```python
from build123d import *

# Parameters (mm, degrees)
SKETCH1_W          = 71
SKETCH1_H          = 7
EXTRUDE1_DEPTH     = 5.5
SKETCH2_W          = 65
SKETCH2_H          = 2.766320183
CUT_EXTRUDE1_DEPTH = 7.5
SKETCH3_W          = 63
SKETCH3_H          = 2
EXTRUDE2_DEPTH     = 5.5
SKETCH4_W          = 49.4
SKETCH4_H          = 2
SKETCH4_W_2        = 12.5
CUT_EXTRUDE2_DEPTH = 2.9
FILLET1_R          = 2
EXTRUDE3_START     = 1.955331485
EXTRUDE3_DEPTH     = 2.978778395
EXTRUDE3_START_2   = -35.5
EXTRUDE3_2_DEPTH   = 71


with BuildPart() as part:
    # Sketch1 → Extrude1 (new body)
    with BuildSketch(Plane(origin=(0, 0, 0), x_dir=(1, 0, 0), z_dir=(0, 1, 0))):
        Rectangle(SKETCH1_W, SKETCH1_H)
    extrude(amount=EXTRUDE1_DEPTH)

    # Sketch2 → Cut-Extrude1 (cut)
    with BuildSketch(Plane(origin=(0, 5.5, 0), x_dir=(-1, 0, 0), z_dir=(0, 1, 0))):
        with Locations((0, 3.383160092)):
            Rectangle(SKETCH2_W, SKETCH2_H)
    extrude(amount=-CUT_EXTRUDE1_DEPTH, mode=Mode.SUBTRACT)

    # Sketch3 → Extrude2 (add)
    with BuildSketch(Plane(origin=(0, 5.5, 0), x_dir=(-1, 0, 0), z_dir=(0, 1, 0))):
        with Locations((0, -4.5)):
            Rectangle(SKETCH3_W, SKETCH3_H)
    extrude(amount=-EXTRUDE2_DEPTH)

    # Sketch4 → Cut-Extrude2 (cut)
    with BuildSketch(Plane(origin=(0, 5.5, 0), x_dir=(-1, 0, 0), z_dir=(0, 1, 0))):
        with Locations((-6.8, -4.5)):
            Rectangle(SKETCH4_W, SKETCH4_H)
        with Locations((25.25, -4.5)):
            Rectangle(SKETCH4_W_2, SKETCH4_H)
    extrude(amount=-CUT_EXTRUDE2_DEPTH, mode=Mode.SUBTRACT)

    # Fillet1
    fillet1_edges = [part.edges().sort_by_distance(p)[0] for p in [
        (-18.45, 5.5, -5.5),
    ]]
    fillet(fillet1_edges, radius=FILLET1_R)

    # Extrude3: read off the stored shape, not the designer's step
    # Extrude3 outline → Extrude3 (cut)
    with BuildSketch(Plane(origin=(0, 0, 0), x_dir=(1, 0, 0), z_dir=(0, 1, 0)).offset(EXTRUDE3_START)):
        Polygon((-19, 3.5), (-34.670728733, 3.5), (-35.248026649, 0.655722687), (35.324444086, 0.655722687), (34.74714617, 3.5), (-17.9, 3.5), (-18.45, 0.790216232), align=None)
    extrude(amount=EXTRUDE3_DEPTH, mode=Mode.SUBTRACT)

    # Extrude3 2 outline → Extrude3 2 (add)
    with BuildSketch(Plane.YZ.offset(EXTRUDE3_START_2)):
        Polygon((1.955331485, -3.5), (3.133469723, -3.5), (1.955331485, -0.655722687), align=None)
    extrude(amount=EXTRUDE3_2_DEPTH)


solid = part.part
```
Input: part model. Units: mm. Frame: model coordinates. A direction names the side the tool comes from. Coordinates: 2 decimals unless noted, no trailing zeros. Write each loop counter-clockwise with the first axis right and the second up, starting at its lowest first coordinate (ties: lowest second). Pieces come first, ordered by that corner, then holes. Notation, with made-up numbers: (76, -20) -> (106, -20) arc R19 ccw to (106, 9) -> close; hole circle Ø8 at (37, -6). An arc over 180 degrees is marked (long way). Write each question's results on one line, items separated by ' | '.
Item 1: Mould query, pull axis Z, two halves, no side actions, for faces 1 (the flat face through (0, 3, -0.656)), 2 (the flat face through (0, 1, -5.5)), 3 (the flat face through (-17.9, 4, -5)). Classes: +Z half, -Z half, draft (parallel to the pull), parting line (faces both ways), or undercut.
Conclusion:
face 1: undercut | face 2: -Z half | face 3: draft
Item 2: Section query B-B on x = 17. Return loops of the section in (y, z), plus the area to 3 significant figures.
Conclusion:
outline: (0, -5.5) -> (2.6, -5.5) -> (2.6, -3.5) -> (3.13, -3.5) -> (1.96, -0.66) -> (4.93, -0.66) -> (4.93, -3.5) -> (5.5, -3.5) -> (5.5, 2) -> (0, 2) -> close | area: 28.7 mm^2
Item 3: Section query C-C on y = 1.1. Return loops of the section in (x, z), plus the area to 4 significant figures.
Conclusion:
outline: (-35.5, -3.5) -> (-31.5, -3.5) -> (-31.5, -5.5) -> (31.5, -5.5) -> (31.5, -3.5) -> (35.5, -3.5) -> (35.5, 3.5) -> (32.5, 3.5) -> (32.5, 2) -> (-32.5, 2) -> (-32.5, 3.5) -> (-35.5, 3.5) -> close | area: 525.5 mm^2
Item 4: Material intervals for probe 1 along X at (y, z) = (1.5, 2.75); probe 2 along X at (y, z) = (3.8, -1.5); probe 3 along Y at (x, z) = (-2, -0.75), sorted ascending.
Conclusion:
probe 1: x = -35.5 to -32.5, 32.5 to 35.5 | probe 2: x = -35.5 to -35.08, -18.59 to -18.31, 35.15 to 35.5 | probe 3: y = 0 to 1.99, 4.93 to 5.5
Item 5: Pin query (flat end, axial travel): pin 1 Ø1 at (x, z) = (-23.5, -4.5) entering from +Y; pin 2 Ø0.6 at (y, z) = (3.5, -4) entering from -X; pin 3 Ø1 at (y, z) = (1.5, -4.5) entering from -X. Return the tip coordinate at first contact, or that it passes through.
Conclusion:
pin 1: stops at y = 2.6 | pin 2: stops at x = -19 | pin 3: stops at x = -31.5
Item 6: Section query A-A on z = 2.75. Return loops of the section in (x, y), plus the area to 3 significant figures.
Conclusion:
outline: (-35.5, 0) -> (-32.5, 0) -> (-32.5, 5.5) -> (-35.5, 5.5) -> close; (32.5, 0) -> (35.5, 0) -> (35.5, 5.5) -> (32.5, 5.5) -> close | area: 33.0 mm^2
Item 7: Section query D-D on z = -2.75. Return loops of the section in (x, y), plus the area to 3 significant figures.
Conclusion:
outline: (-35.5, 0) -> (35.5, 0) -> (35.5, 5.5) -> (-35.5, 5.5) -> close; hole (-34.82, 2.82) -> (-18.85, 2.82) -> (-18.85, 4.93) -> (-34.82, 4.93) -> close; hole (-18.05, 2.82) -> (34.9, 2.82) -> (34.9, 4.93) -> (-18.05, 4.93) -> close | area: 245 mm^2
Item 8: Set-up query: faces 4 (the flat face through (7, 2.6, -4)), 5 (the flat face through (-32.5, 3, 3)), 6 (the flat face through (35.04, 3.75, -2.06)), 7 (the flat face through (-31.5, 1, -5)). Return all of +Z, -Z, +X, -X, +Y, -Y with unobstructed straight access to the full face (end or side cutting, diameter ignored); none if empty.
Conclusion:
face 4: -Z, +X, +Y | face 5: +Z, +Y, -Y | face 6: none | face 7: -Z, -X, +Y, -Y
